Build history of the part. All positions in model axes, mm. Face numbers are marked on the shaded views. A direction names the side the tool comes from. Round coordinates to 2 decimals unless told otherwise and drop trailing zeros. Write each loop counter-clockwise with the first axis right and the second up, starting at its lowest first coordinate (ties: lowest second). Pieces come first, ordered by that corner, then holes. Notation, with made-up numbers: (85.5, -5) - (93.5, -5) arc R14 ccw to (93.5, 4) - close; hole circle Ø2 at (42, -4.5). An arc over 180 degrees is marked (long way). Answer as a JSON object with one key per item and string values. Group by question number.
Item 1: Slice it at B-B, the plane z = 5.25. List the corners of the cut face in (x, y), then the cut area to 3 significant figures.
Item 2: Slice it at A-A, the plane x = 12.5. List the corners of the cut face in (y, z).
Item 3: Two-plate mould, pull along X, no slides. Class the marked faces 1, 2 and 3: +X half, -X half, draft (parallel to the pull), parting line (faces both ways), or undercut.
Item 4: Which spindle directions (+Z, -Z, +X, -X, +Y, -Y) get a long thin tool onto all of the face, cutting with end or side? Do the marked faces 4, 5 and 6. Say none if no direction does.
Item 5: Slice it at C-C, the plane z = 9. List the corners of the cut face in (x, y), then the cut area to 3 significant figures.
Item 6: Flat gauge pins, fed straight in: pin 1 (2.5 mm diameter, centred on x = 0, z = 5.5, fed in from +Y); pin 2 (1.5 mm diameter, centred on x = 2, y = -3.5, fed in from +Z); pin 3 (3.5 mm diameter, centred on x = -1, z = 5, fed in from -Y); pin 4 (4 mm diameter, centred on y = -5.5, z = 11, fed in from -X). Where does each tip first touch, or does it go through?
Item 7: Probe line 1 (Y direction, x = 12.5, z = 15.2); line 2 (Z direction, x = 3, y = 6.5); line 3 (Z direction, x = -2.5, y = 2.5). List the from-to ranges inside material, lowest first. Write a range as from..to.
Item 8: Slice it at D-D, the plane y = -8.5. List the corners of the cut face in (x, z).
from build123d import *

# Parameters (mm, degrees)
SKETCH1_W           = 45
SKETCH1_H           = 20
BOSS_EXTRUDE1_DEPTH = 3.5
SKETCH2_R           = 8
BOSS_EXTRUDE2_DEPTH = 12
SKETCH3_R           = 6
CUT_EXTRUDE1_DEPTH  = 0.5
FILLET1_R           = 0.25
BOSS_EXTRUDE3_DEPTH = 3.5
FILLET2_R           = 0.25


with BuildPart() as part:
    # Sketch1 → Boss-Extrude1 (new body)
    with BuildSketch(Plane.XY):
        Rectangle(SKETCH1_W, SKETCH1_H)
    extrude(amount=BOSS_EXTRUDE1_DEPTH)

    # Sketch2 → Boss-Extrude2 (add)
    with BuildSketch(Plane.XY.offset(3.5)):
        with Locations((12.5, 0)):
            Circle(SKETCH2_R)
        with Locations((-12.5, 0)):
            Circle(SKETCH2_R)
    extrude(amount=BOSS_EXTRUDE2_DEPTH)

    # Sketch3 → Cut-Extrude1 (cut)
    with BuildSketch(Plane.XY.offset(15.5)):
        with Locations((-12.5, 0)):
            Circle(SKETCH3_R)
        with Locations((12.5, 0)):
            Circle(SKETCH3_R)
    extrude(amount=-CUT_EXTRUDE1_DEPTH, mode=Mode.SUBTRACT)

    # Fillet1
    fillet1_edges = [part.edges().sort_by_distance(p)[0] for p in [
        (4.5, 0, 15.5),
        (-20.5, 0, 15.5),
    ]]
    fillet(fillet1_edges, radius=FILLET1_R)

    # Sketch4 → Boss-Extrude3 (add)
    with BuildSketch(Plane.XY.offset(3.5)):
        with BuildLine():
            Line((-3.25, 9.25), (3.25, 9.25))
            ThreePointArc((3.25, 9.25), (5, 7.5), (3.25, 5.75))
            Line((3.25, 5.75), (-3.25, 5.75))
            ThreePointArc((-3.25, 5.75), (-5, 7.5), (-3.25, 9.25))
        make_face()
    extrude(amount=BOSS_EXTRUDE3_DEPTH)

    # Fillet2
    fillet2_edges = [part.edges().sort_by_distance(p)[0] for p in [
        (-5, 7.5, 7),
        (0, 5.75, 7),
        (5, 7.5, 7),
        (0, 9.25, 7),
    ]]
    fillet(fillet2_edges, radius=FILLET2_R)


solid = part.part
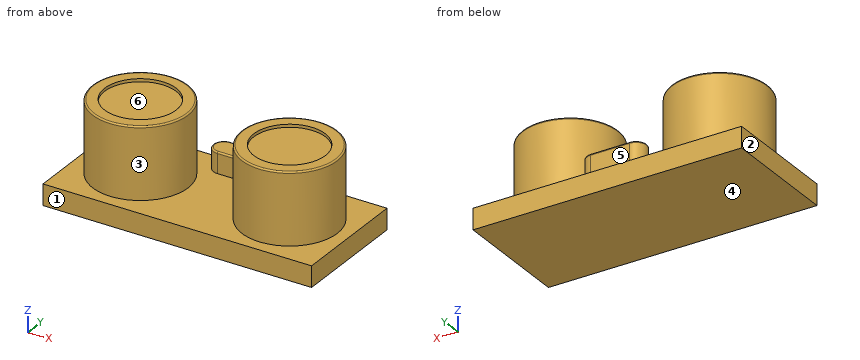
Geometry says:
{
 "1": {"outline": "circle Ø16 at (-12.5, 0); (-3.25, 5.75) - (3.25, 5.75) arc R1.75 ccw to (3.25, 9.25) - (-3.25, 9.25) arc R1.75 ccw to start; circle Ø16 at (12.5, 0)", "area": "434 mm^2"},
 "2": {"outline": "(-10, 0) - (10, 0) - (10, 3.5) - (8, 3.5) - (8, 15.25) arc R0.25 ccw to (7.75, 15.5) - (6, 15.5) - (6, 15) - (-6, 15) - (-6, 15.5) - (-7.75, 15.5) arc R0.25 ccw to (-8, 15.25) - (-8, 3.5) - (-10, 3.5) - close"},
 "3": {"face 1": "draft", "face 2": "-X half", "face 3": "undercut"},
 "4": {"face 4": "-Z, +X, -X, +Y, -Y", "face 5": "+Z, +X, -X, +Y", "face 6": "+Z"},
 "5": {"outline": "circle Ø16 at (-12.5, 0); circle Ø16 at (12.5, 0)", "area": "402 mm^2"},
 "6": {"pin 1": "stops at y = 9.25", "pin 2": "stops at z = 3.5", "pin 3": "stops at y = -10", "pin 4": "stops at x = -19.69"},
 "7": {"line 1": "y = -8..-6, 6..8", "line 2": "z = 0..7", "line 3": "z = 0..3.5"},
 "8": {"outline": "(-22.5, 0) - (22.5, 0) - (22.5, 3.5) - (-22.5, 3.5) - close"}
}
